Design review of the part shown in the three views and the two pictorial views. Dimensions are in mm from the part's minimum x, y and z. Round coordinates to 2 decimals unless told otherwise and drop trailing zeros. Write each loop counter-clockwise with the first axis right and the second up, starting at its lowest first coordinate (ties: lowest second). Pieces come first, ordered by that corner, then holes. Notation, with made-up numbers: (31, 81) - (87, 81) arc R13 ccw to (87, 102) - close; hole circle Ø7 at (9.25, 71.5). An arc over 180 degrees is marked (long way). One line per item, written item: value. Start each with the question number.
Q1. Add section B-B on y = 20. Write out the cut boundary in (x, z), and give its area (3 significant figures).
Q2. Add section D-D on x = 12.5. Write out the cut boundary in (y, z), and give its area (3 significant figures).
Q3. For probe 1 along Y at (x, z) = (25, 1); probe 2 along Y at (x, z) = (42.8, 1.7); probe 3 along X at (y, z) = (19, 0.95), list the stretches that pass through material, from the lowest coordinate up.
Q4. Add section A-A on y = 35. Write out the cut boundary in (x, z), and give its area (3 significant figures).
Q5. Clearance check with a flat-ended pin moving along its axis: pin 1 Ø13 at (x, y) = (10, 35) entering from -Z. State where the tip first meets the part, or that it passes through.
Q6. Add section C-C on z = 0.7. Give the number of separate pieces and of enclosed holes in the cut face, and give its area (3 significant figures).
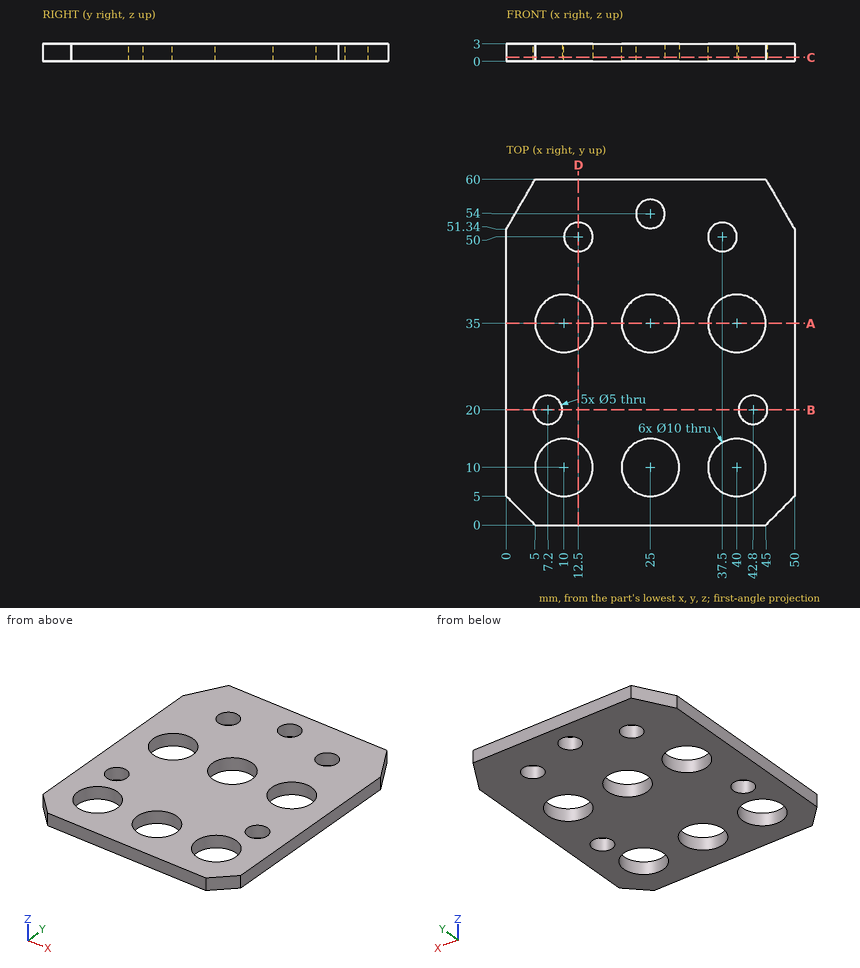
Result set:
1. outline: (0, 0) - (4.7, 0) - (4.7, 3) - (0, 3) - close; (9.7, 0) - (40.3, 0) - (40.3, 3) - (9.7, 3) - close; (45.3, 0) - (50, 0) - (50, 3) - (45.3, 3) - close
1. area: 120 mm^2
2. outline: (0, 0) - (5.67, 0) - (5.67, 3) - (0, 3) - close; (14.33, 0) - (30.67, 0) - (30.67, 3) - (14.33, 3) - close; (39.33, 0) - (47.5, 0) - (47.5, 3) - (39.33, 3) - close; (52.5, 0) - (60, 0) - (60, 3) - (52.5, 3) - close
2. area: 113 mm^2
3. probe 1: y = 0 to 5, 15 to 30, 40 to 51.5, 56.5 to 60
3. probe 2: y = 0 to 5.86, 14.14 to 17.5, 22.5 to 30.86, 39.14 to 60
3. probe 3: x = 0 to 4.91, 9.49 to 40.51, 45.09 to 50
4. outline: (0, 0) - (5, 0) - (5, 3) - (0, 3) - close; (15, 0) - (20, 0) - (20, 3) - (15, 3) - close; (30, 0) - (35, 0) - (35, 3) - (30, 3) - close; (45, 0) - (50, 0) - (50, 3) - (45, 3) - close
4. area: 60.0 mm^2
5. pin 1: stops at z = 0
6. separate pieces: 1
6. enclosed holes: 11
6. area: 2,360 mm^2
